```python
from build123d import *

# Parameters (mm, degrees)
F0_W     = 2
F0_H     = 1.5
F0_H_2   = 20
F0_W_2   = 11
F0_W_3   = 7
F1_DEPTH = 3
F3_DEPTH = 26.5
F5_R     = 2
F6_DEPTH = 27
F7_R     = 0.75
F8_DEPTH = 0.5
F9_R     = 0.49999


# Not quite as in the source:
# - a fillet or chamfer is up to 0.001 mm smaller than in the source, because OpenCascade refuses the exact size


with BuildPart() as f1:
    # F0 (on Top) → F1 (new body)
    with BuildSketch(Plane.XY):
        Polygon((-1.7407407407, 9.2222222222), (5.2592592593, 9.2222222222), (16.2592592593, 9.2222222222), (16.2592592593, 10.7222222222), (18.2592592593, 10.7222222222), (18.2592592593, 9.2222222222), (20.2592592593, 9.2222222222), (20.2592592593, 14.2222222222), (-16.7407407407, 14.2222222222), (-16.7407407407, 9.2222222222), (-14.7407407407, 9.2222222222), (-14.7407407407, 10.7222222222), (-12.7407407407, 10.7222222222), (-12.7407407407, 9.2222222222), align=None)
        Polygon((16.2592592593, -10.7777777778), (5.2592592593, -10.7777777778), (-1.7407407407, -10.7777777778), (-12.7407407407, -10.7777777778), (-12.7407407407, -12.2777777778), (-14.7407407407, -12.2777777778), (-14.7407407407, -10.7777777778), (-16.7407407407, -10.7777777778), (-16.7407407407, -15.7777777778), (20.2592592593, -15.7777777778), (20.2592592593, -10.7777777778), (18.2592592593, -10.7777777778), (18.2592592593, -12.2777777778), (16.2592592593, -12.2777777778), align=None)
        with Locations((17.2592592593, 9.9722222222)):
            Rectangle(F0_W, F0_H)
        with Locations((17.2592592593, -0.7777777778)):
            Rectangle(F0_W, F0_H_2)
        with Locations((-13.7407407407, -0.7777777778)):
            Rectangle(F0_W, F0_H_2)
        with Locations((-13.7407407407, 9.9722222222)):
            Rectangle(F0_W, F0_H)
        with Locations((17.2592592593, -11.5277777778)):
            Rectangle(F0_W, F0_H)
        with Locations((-13.7407407407, -11.5277777778)):
            Rectangle(F0_W, F0_H)
        with Locations((-7.2407407407, -0.7777777778)):
            Rectangle(F0_W_2, F0_H_2)
        with Locations((1.7592592593, -0.7777777778)):
            Rectangle(F0_W_3, F0_H_2)
        with Locations((10.7592592593, -0.7777777778)):
            Rectangle(F0_W_2, F0_H_2)
    extrude(amount=F1_DEPTH)

    # F5 (on face) → F6 (join)
    with BuildSketch(Plane(origin=(0, 14.2222222222, 0), x_dir=(-1, 0, 0), z_dir=(0, 1, 0))):
        with Locations((-1.7592592593, -1.4)):
            Circle(F5_R)
    extrude(amount=-F6_DEPTH)

    # F7 (on face) → F8 (join)
    with BuildSketch(Plane(origin=(0, 0, 0), x_dir=(1, 0, 0), z_dir=(0, 0, -1))):
        with Locations((-7.2407407407, 13.2777777778)):
            Circle(F7_R)
        with Locations((10.7592592593, 13.2777777778)):
            Circle(F7_R)
    extrude(amount=F8_DEPTH)

    # F9 (radius 0.5 in the source; OpenCascade refuses exactly that, so slightly less here)
    f9_edges = [f1.edges().sort_by_distance(p)[0] for p in [
        (10.009259, -13.277778, -0.5),
        (-7.990741, -13.277778, -0.5),
    ]]
    fillet(f9_edges, radius=F9_R)


with BuildPart() as f3:
    # F2 (on face) → F3 (new body)
    with BuildSketch(Plane(origin=(0, 14.2222222222, 0), x_dir=(-1, 0, 0), z_dir=(0, 1, 0))):
        with BuildLine():
            ThreePointArc((-1.3930631716, 0), (-0.7580650487, -3.223722123), (1.975, -1.4))
            ThreePointArc((1.975, -1.4), (1.823722123, -0.6419349513), (1.3930631716, 0))
            Line((1.3930631716, 0), (-1.3930631716, 0))
        make_face()
    extrude(amount=-F3_DEPTH)


solid = f1.part
```
Source: CAD feature listing. Evaluate the final solid. Frame: model axes, mm. A direction names the side the tool comes from. Round coordinates to 2 decimals unless told otherwise and drop trailing zeros. Loops run counter-clockwise (first coordinate to the right, second up) from the corner with the lowest first, then second, coordinate; pieces in that order, holes last. Notation, with made-up numbers: M 36,57.5 L 67,57.5 A23 ccw 67,67.5 Z; hole C 12,86.5 d1. An arc over 180 degrees is marked long. Use a Markdown table: item, result. Add a question column.
1. Cut plane A-A, the plane z = 2.25. Output: boundary loops of the cut face in (x, y).
2. Contact query for flat-ended pins moving along their axis: pin 1 (9 mm diameter, centred on x = 8, y = 1.5, fed in from -Z); pin 2 (3.5 mm diameter, centred on y = 2, z = 2, fed in from +X); pin 3 (2.5 mm diameter, centred on y = -3, z = 1, fed in from -X). Output: stop coordinate, or through.
3. Ray query, line 1 along Y through (x, z) = (0.5, -2.5); line 2 along X through (y, z) = (-8, 1.5); line 3 along X through (y, z) = (12, -1.5). Return the intervals inside material, ascending. Write a range as [from, to].
4. Set-up query: faces 1 (the flat face through (20.259, 12, 1)), 2 (the flat face through (-16, 9.222, 1)), 3 (the flat face through (18.259, -1, 1)). Return all of +Z, -Z, +X, -X, +Y, -Y with unobstructed straight access to the full face (end or side cutting, diameter ignored); none if empty.
5. Cut plane C-C, the plane x = 7. Output: boundary loops of the cut face in (y, z).
6. Cut plane B-B, the plane y = -1.5. Output: boundary loops of the cut face in (x, z).
7. Cut plane D-D, the plane z = -1.4. Output: boundary loops of the cut face in (x, y).
Solution:
| question | item | result |
|---|---|---|
| 1 | outline | M -16.74,-15.78 L 20.26,-15.78 L 20.26,-10.78 L 18.26,-10.78 L 18.26,9.22 L 20.26,9.22 L 20.26,14.22 L -16.74,14.22 L -16.74,9.22 L -14.74,9.22 L -14.74,-10.78 L -16.74,-10.78 Z |
| 2 | pin 1 | stops at z = -2.38 |
| 2 | pin 2 | stops at x = 18.26 |
| 2 | pin 3 | stops at x = -14.74 |
| 3 | line 1 | y = [-12.78, 14.22] |
| 3 | line 2 | x = [-14.74, 18.26] |
| 3 | line 3 | x = [-0.24, 3.76] |
| 4 | face 1 | +Z, -Z, +X, +Y, -Y |
| 4 | face 2 | +Z, -Z, -X |
| 4 | face 3 | +Z, -Z, +X |
| 5 | outline | M -15.78,0 L 14.22,0 L 14.22,3 L -15.78,3 Z |
| 6 | outline | M -14.74,0 L 0.33,0 A2 ccw long 3.19,0 L 18.26,0 L 18.26,3 L -14.74,3 Z |
| 7 | outline | M -0.24,-12.78 L 3.76,-12.78 L 3.76,14.22 L -0.24,14.22 Z |
